For this review, take the finished solid that the model builds, in its own axes (mm). A direction names the side the tool comes from. Round coordinates to 2 decimals unless told otherwise and drop trailing zeros. Order: outer loops, then holes, each group sorted by start corner. A loop starts at its lowest first (then second) coordinate and runs counter-clockwise, first axis right, second up. Notation, with made-up numbers: (-32, 70.5) - (-12, 70.5) arc R19 cw to (-12, 82.5) - close; hole circle Ø4 at (-7.5, -10). An arc over 180 degrees is marked (long way). One line per question, with ' | ' between items.
```python
from build123d import *

# Parameters (mm, degrees)
F2_W     = 10.16
F2_H     = 17.78
F3_DEPTH = 12.7
F4_R     = 5.08
F5_R     = 3.777996
F6_DEPTH = 25.4


with BuildPart() as f1:
    # F0 (on Top) → F1 (revolve)
    with BuildSketch(Plane.XY):
        Polygon((0, 0), (38.1, 0), (38.1, 18.348159), (30.580265, 22.860002), (38.1, 26.770264), (38.1, 43.18), (0, 43.18), align=None)
    revolve(axis=Axis((0, 21.59, 0), (0, 1, 0)))

    # F2 (on face) → F3 (join)
    with BuildSketch(Plane(origin=(0, 43.18, 0), x_dir=(-1, 0, 0), z_dir=(0, 1, 0))):
        Rectangle(F2_W, F2_H)
    extrude(amount=F3_DEPTH)

    # F4
    f4_edges = [f1.edges().sort_by_distance(p)[0] for p in [
        (0, 55.88, 8.89),
        (0, 55.88, -8.89),
    ]]
    fillet(f4_edges, radius=F4_R)

    # F5 (on face) → F6 (cut)
    with BuildSketch(Plane.YZ.offset(5.08)):
        with Locations((48.678428, 0)):
            Circle(F5_R)
    extrude(amount=-F6_DEPTH, mode=Mode.SUBTRACT)


solid = f1.part
```
(1) We need section C-C on x = 0. State the section outline as (y, z) points.
Output values:
outline: (0, -38.1) - (18.35, -38.1) - (22.86, -30.58) - (26.77, -38.1) - (43.18, -38.1) - (43.18, -8.89) - (50.8, -8.89) arc R5.08 ccw to (55.88, -3.81) - (55.88, 3.81) arc R5.08 ccw to (50.8, 8.89) - (43.18, 8.89) - (43.18, 38.1) - (26.77, 38.1) - (22.86, 30.58) - (18.35, 38.1) - (0, 38.1) - close; hole circle Ø7.56 at (48.68, 0)
(2) We need section D-D on y = 11. State the section outline as (x, z) points.
Output values:
outline: circle Ø76.2 at (0, 0)
(3) We need section B-B on z = 0. State the section outline as (x, y) points.
Output values:
outline: (-38.1, 0) - (38.1, 0) - (38.1, 18.35) - (30.58, 22.86) - (38.1, 26.77) - (38.1, 43.18) - (5.08, 43.18) - (5.08, 44.9) - (-5.08, 44.9) - (-5.08, 43.18) - (-38.1, 43.18) - (-38.1, 26.77) - (-30.58, 22.86) - (-38.1, 18.35) - close; (-5.08, 52.46) - (5.08, 52.46) - (5.08, 55.88) - (-5.08, 55.88) - close
(4) For faces 4 (the flat face through (5.08, 52.3, 1.9)), 5 (the flat face through (0, 47, -8.89)), 6 (the flat face through (0, 55.88, 0)), 7 (the conical face through (-6.731, 23.105, 30.312)), 8 (the flat face through (0, 47, 8.89)), list the 3-axis set-ups (+Z, -Z, +X, -X, +Y, -Y) from which the entire face can be reached by the end or side of a thin tool; tool diameter is ignored.
Output values:
face 4: +Z, -Z, +X, +Y | face 5: -Z, +X, -X, +Y | face 6: +Z, -Z, +X, -X, +Y | face 7: none | face 8: +Z, +X, -X, +Y
(5) Mouldability with a two-part tool opening along Z and no side actions: class faces 1 (the cylindrical face through (-0.071, 54.352, 7.441)), 2 (the cylindrical face through (0.071, 44.904, 0.166)), 3 (the flat face through (-5.08, 52.3, 1.9)) as released by +Z, released by -Z, zero draft, split by the parting line, or undercut.
Output values:
face 1: released by +Z | face 2: undercut | face 3: zero draft
(6) Insertion check: pin 1 (8.5 mm diameter, centred on x = -1, y = 46.5, fed in from -Z); pin 2 (4 mm diameter, centred on x = -1, y = 47.5, fed in from +Z); pin 3 (8 mm diameter, centred on x = -22.5, y = 36, fed in from +Z). Each pin has a flat end and moves straight along its axis. Give the tip position at first contact, or say it passes through.
Output values:
pin 1: z = -38.1 | pin 2: z = 8.89 | pin 3: z = 33.31
(7) For probe 1 along Y at (x, z) = (-31.5, -18); probe 2 along Y at (x, z) = (-24, 24.5); probe 3 along Y at (x, z) = (-25.5, 0.5), list the stretches that pass through material, from the lowest coordinate up. Write a range as [from, to].
Output values:
probe 1: [0, 19.44], [25.82, 43.18] | probe 2: [0, 20.63], [24.79, 43.18] | probe 3: [0, 43.18]
(8) We need section A-A on y = 47.5. State the section outline as (x, z) points.
Output values:
outline: (-5.08, -8.89) - (5.08, -8.89) - (5.08, -3.59) - (-5.08, -3.59) - close; (-5.08, 3.59) - (5.08, 3.59) - (5.08, 8.89) - (-5.08, 8.89) - close
